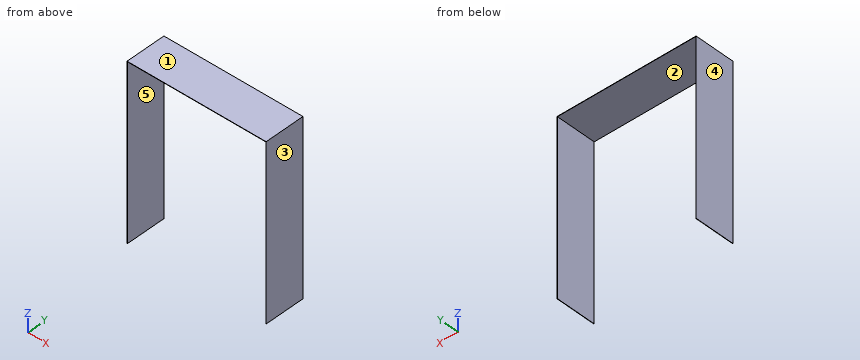
from build123d import *

# Parameters (mm, degrees)
TOPPING_PLINT_U_1_START = 10
TOPPING_PLINT_U_1_DEPTH = 190


with BuildPart() as part:
    # Sketch1 → TOPPING_plint_U_1 (new body)
    with BuildSketch(Plane(origin=(0, 0, 0), x_dir=(1, 0, 0), z_dir=(0, 1, 0)).offset(TOPPING_PLINT_U_1_START)):
        Polygon((20, 800), (20, -20), (680, -20), (680, 800), (678.5, 800), (678.5, -18.5), (21.5, -18.5), (21.5, 800), align=None)
    extrude(amount=TOPPING_PLINT_U_1_DEPTH)


solid = part.part
The model under review builds one solid part; all positions refer to its coordinate system, in mm. Face numbers are marked on the shaded views. A direction names the side the tool comes from. Give positions to 0.01 mm unless a question says otherwise; leave off trailing zeros. Order: outer loops, then holes, each group sorted by start corner. A loop starts at its lowest first (then second) coordinate and runs counter-clockwise, first axis right, second up. Notation, with made-up numbers: M 62,32.25 L 100,32.25 A24 ccw 100,43.25 Z; hole C 8,24 d10. An arc over 180 degrees is marked long. Answer in a Markdown table with one row per item. Add a question column.
1. Mouldability with a two-part tool opening along X and no side actions: class the marked faces 1, 2 and 3 as released by +X, released by -X, zero draft, split by the parting line, or undercut.
2. Add section B-B on y = 143. State the section outline as (x, z) points, plus the area to 3 significant figures.
3. To check wall thickness, follow line 1 along X through (y, z) = (155.5, -511); line 2 along Z through (x, y) = (538.5, 107). State the ranges of each line that lie inside material, in increasing order.
4. Machinability: for the marked faces 4 and 5, which of the approach directions +Z, -Z, +X, -X, +Y, -Y give a long, thin tool a straight path to every point of the face, cutting with its end or side? Answer none if there is none.
5. Add section A-A on z = -490. State the section outline as (x, y) points.
6. For pin 1 Ø12 at (x, y) = (321, 132) entering from -Z, flat-tipped, find the tip position at first contact; note if it passes through.
7. Add section C-C on x = 126. State the section outline as (y, z) points, plus the area to 3 significant figures.
The answers:
| question | item | result |
|---|---|---|
| 1 | face 1 | zero draft |
| 1 | face 2 | undercut |
| 1 | face 3 | released by +X |
| 2 | outline | M 20,-800 L 21.5,-800 L 21.5,18.5 L 678.5,18.5 L 678.5,-800 L 680,-800 L 680,20 L 20,20 Z |
| 2 | area | 3,450 mm2 |
| 3 | line 1 | 20 to 21.5, 678.5 to 680 |
| 3 | line 2 | 18.5 to 20 |
| 4 | face 4 | +Z, -Z, -X, +Y, -Y |
| 4 | face 5 | -Z, +Y, -Y |
| 5 | outline | M 20,10 L 21.5,10 L 21.5,200 L 20,200 Z; M 678.5,10 L 680,10 L 680,200 L 678.5,200 Z |
| 6 | pin 1 | z = 18.5 |
| 7 | outline | M 10,18.5 L 200,18.5 L 200,20 L 10,20 Z |
| 7 | area | 285 mm2 |
